```python
from build123d import *

# Parameters (mm, degrees)
SKETCH3_W           = 182.88
SKETCH3_H           = 58.42
BOSS_EXTRUDE1_DEPTH = 57.15
SKETCH4_W           = 203.2
SKETCH4_H           = 76.2
BOSS_EXTRUDE2_DEPTH = 2.54
SKETCH5_W           = 177.8
SKETCH5_H           = 53.34
CUT_EXTRUDE1_DEPTH  = 54.61
SKETCH6_R           = 2.7813
CUT_EXTRUDE2_DEPTH  = 53.34
SKETCH7_R           = 3.175
CUT_EXTRUDE3_DEPTH  = 3.54


with BuildPart() as part:
    # Sketch3 → Boss-Extrude1 (new body)
    with BuildSketch(Plane(origin=(0, 0, 0), x_dir=(1, 0, 0), z_dir=(0, 1, 0))):
        Rectangle(SKETCH3_W, SKETCH3_H)
    extrude(amount=-BOSS_EXTRUDE1_DEPTH)

    # Sketch4 → Boss-Extrude2 (add)
    with BuildSketch(Plane(origin=(0, 0, 0), x_dir=(1, 0, 0), z_dir=(0, 1, 0))):
        Rectangle(SKETCH4_W, SKETCH4_H)
    extrude(amount=-BOSS_EXTRUDE2_DEPTH)

    # Sketch5 → Cut-Extrude1 (cut)
    with BuildSketch(Plane(origin=(0, 0, 0), x_dir=(1, 0, 0), z_dir=(0, 1, 0))):
        Rectangle(SKETCH5_W, SKETCH5_H)
    extrude(amount=-CUT_EXTRUDE1_DEPTH, mode=Mode.SUBTRACT)

    # Sketch6 → Cut-Extrude2 (cut)
    with BuildSketch(Plane(origin=(0, 0, 0), x_dir=(1, 0, 0), z_dir=(0, 1, 0))):
        with Locations((-95.25, 31.75)):
            Circle(SKETCH6_R)
        with Locations((0, 33.02)):
            Circle(SKETCH6_R)
        with Locations((95.25, 33.02)):
            Circle(SKETCH6_R)
        with Locations((95.25, -33.02)):
            Circle(SKETCH6_R)
        with Locations((0, -33.02)):
            Circle(SKETCH6_R)
        with Locations((-95.25, -31.75)):
            Circle(SKETCH6_R)
    extrude(amount=-CUT_EXTRUDE2_DEPTH, mode=Mode.SUBTRACT)

    # Sketch7 → Cut-Extrude3 (cut, through all)
    with BuildSketch(Plane(origin=(0, -54.61, 0), x_dir=(1, 0, 0), z_dir=(0, 1, 0))):
        with Locations((-63.5, 12.7)):
            Circle(SKETCH7_R)
        with Locations((-50.8, 0)):
            Circle(SKETCH7_R)
        with Locations((-63.5, -12.7)):
            Circle(SKETCH7_R)
        with Locations((-76.2, 0)):
            Circle(SKETCH7_R)
    extrude(amount=-CUT_EXTRUDE3_DEPTH, mode=Mode.SUBTRACT)


solid = part.part
```
Can you work these out from the model? Positions are in its coordinate system, mm. A direction names the side the tool comes from. Coordinates: 2 decimals unless noted, no trailing zeros. Loops run counter-clockwise (first coordinate to the right, second up) from the corner with the lowest first, then second, coordinate; pieces in that order, holes last. Notation, with made-up numbers: (23.5, -29) -> (80.5, -29) arc R16 cw to (80.5, -6) -> close; hole circle Ø3 at (83, 21.5). An arc over 180 degrees is marked (long way). Put each result on its own line as item: value. Start each with the question number.
Q1. If I drill on line 1 (X direction, y = -56.2, z = 0) (3 decimals); line 2 (Z direction, x = -0.5, y = -31.5); line 3 (X direction, y = -34, z = -11.5), over which ranges is the centre line in solid material (lowest first)? Write a range as [from, to].
Q2. I'm going to push flat-ended pins straight in: P1, Ø2, axis at x = -44, z = 0.5, coming from the +Y side; P2, Ø1.5, axis at y = -20.5, z = 9, coming from the -X side; P3, Ø1.5, axis at y = -18, z = 26, coming from the +X side; P4, Ø4, axis at x = -50.8, z = 0, coming from the +Y side. Where does each tip first touch, or does it pass through?
Q3. Thinking about a two-plate mould opening in X: for faces 1 (the face through (-1, -29, 29.21)), 2 (the face through (-91.44, -29, 0)), 3 (the face through (91.44, -29, 0)), 4 (the face through (-53.97, -55.86, -0.14)), which applies, pulls with the +X half, pulls with the -X half, needs draft (parallel to the pull), parting line crosses it, or undercut?
Q4. I want a section at B-B (x = 95.25). Write out the boundary of the cut face in (y, z).
Q5. I want a section at C-C (x = -50.8). Write out the boundary of the cut face in (y, z) (3 decimals).
Q6. I want a section at A-A (z = -12.7). Write out the boundary of the cut face in (x, y) (3 decimals).
Q7. For faces 5 (the face through (-88.9, -27, 0)), 6 (the face through (-73.17, -55.86, -0.95)), which set-ups out of +Z, -Z, +X, -X, +Y, -Y let a thin tool reach every point of the face, with its end or its side?
Q8. I want a section at D-D (y = -42). Write out the boundary of the cut face in (x, z), plus the area to 3 significant figures.
Taken from the geometry:
1. line 1: x = [-91.44, -79.375], [-73.025, -53.975], [-47.625, 91.44]
1. line 2: z = [-29.21, -26.67], [26.67, 29.21]
1. line 3: x = [-91.44, -88.9], [88.9, 91.44]
2. P1: stops at y = -54.61
2. P2: stops at x = -91.44
2. P3: stops at x = 91.44
2. P4: passes through
3. face 1: needs draft
3. face 2: pulls with the -X half
3. face 3: pulls with the +X half
3. face 4: undercut
4. outline: (-2.54, -38.1) -> (0, -38.1) -> (0, -35.8) -> (-2.54, -35.8) -> close; (-2.54, -30.24) -> (0, -30.24) -> (0, 30.24) -> (-2.54, 30.24) -> close; (-2.54, 35.8) -> (0, 35.8) -> (0, 38.1) -> (-2.54, 38.1) -> close
5. outline: (-57.15, -29.21) -> (-2.54, -29.21) -> (-2.54, -38.1) -> (0, -38.1) -> (0, -26.67) -> (-54.61, -26.67) -> (-54.61, -3.175) -> (-57.15, -3.175) -> close; (-57.15, 3.175) -> (-54.61, 3.175) -> (-54.61, 26.67) -> (0, 26.67) -> (0, 38.1) -> (-2.54, 38.1) -> (-2.54, 29.21) -> (-57.15, 29.21) -> close
6. outline: (-101.6, -2.54) -> (-91.44, -2.54) -> (-91.44, -57.15) -> (-66.675, -57.15) -> (-66.675, -54.61) -> (-88.9, -54.61) -> (-88.9, 0) -> (-101.6, 0) -> close; (-60.325, -57.15) -> (91.44, -57.15) -> (91.44, -2.54) -> (101.6, -2.54) -> (101.6, 0) -> (88.9, 0) -> (88.9, -54.61) -> (-60.325, -54.61) -> close
7. face 5: +Y
7. face 6: +Y, -Y
8. outline: (-91.44, -29.21) -> (91.44, -29.21) -> (91.44, 29.21) -> (-91.44, 29.21) -> close; hole (-88.9, -26.67) -> (88.9, -26.67) -> (88.9, 26.67) -> (-88.9, 26.67) -> close
8. area: 1,200 mm2
